Design review of the part shown in the three views and the two pictorial views. Dimensions are in mm from the part's minimum x, y and z. Round coordinates to 2 decimals unless told otherwise and drop trailing zeros. Loops run counter-clockwise (first coordinate to the right, second up) from the corner with the lowest first, then second, coordinate; pieces in that order, holes last. Notation, with made-up numbers: (-20.75, 50.25) -> (-7.75, 50.25) arc R13 cw to (-7.75, 59.25) -> close; hole circle Ø11 at (-33, 25). An arc over 180 degrees is marked (long way). Return JSON: item names as keys, results as strings. Group by question number.
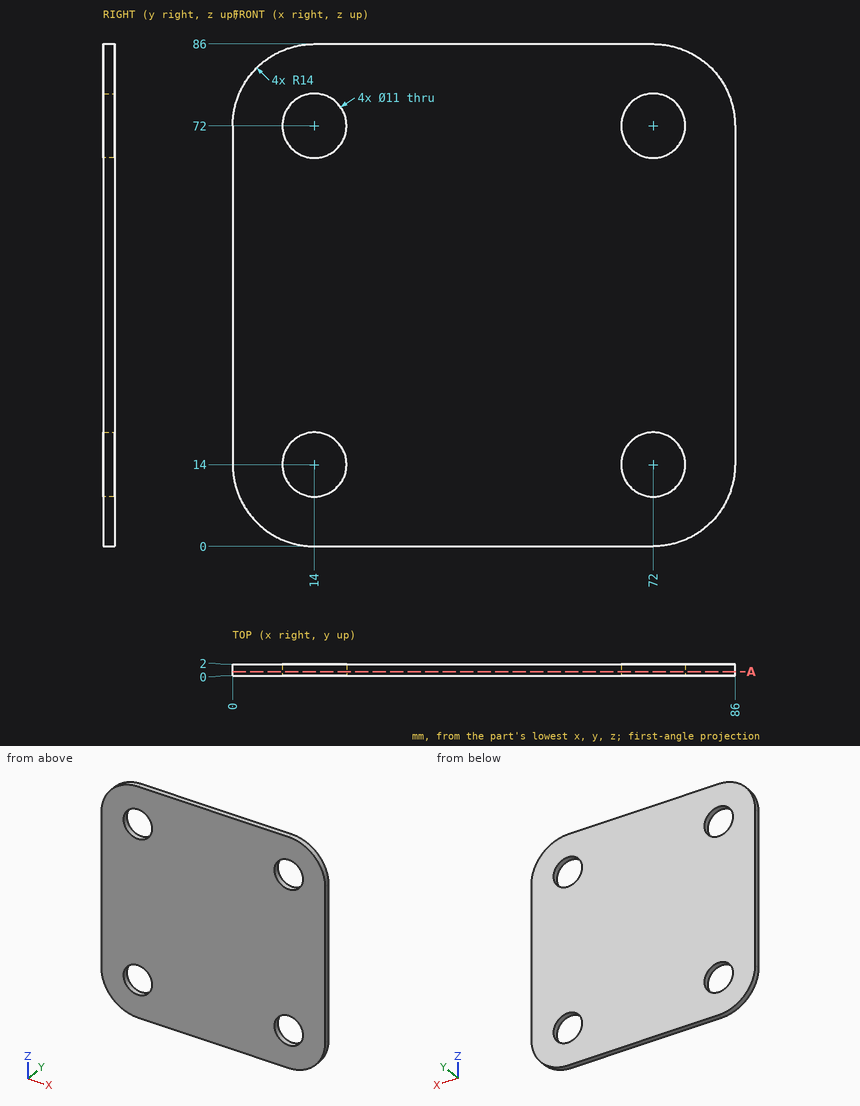
1. Wall thickness on line 1 (X direction, y = 0.85, z = 14); line 2 (Z direction, x = 19, y = 1.85): over which ranges is each line inside the solid? List them lowest first.
2. For P1, Ø10, axis at x = 14, z = 14, coming from the +Y side, flat-tipped, find the tip position at first contact; note if it passes through.
3. We need section A-A, the plane y = 0.75. Write out the cut boundary in (x, z), then the cut area to 3 significant figures.
Check sheet entries:
{
 "1": {"line 1": "x = 0 to 8.5, 19.5 to 66.5, 77.5 to 86", "line 2": "z = 0 to 11.71, 16.29 to 69.71, 74.29 to 86"},
 "2": {"P1": "passes through"},
 "3": {"outline": "(0, 14) arc R14 ccw to (14, 0) -> (72, 0) arc R14 ccw to (86, 14) -> (86, 72) arc R14 ccw to (72, 86) -> (14, 86) arc R14 ccw to (0, 72) -> close; hole circle Ø11 at (14, 14); hole circle Ø11 at (14, 72); hole circle Ø11 at (72, 14); hole circle Ø11 at (72, 72)", "area": "6,850 mm²"}
}
